```python
from build123d import *

# Parameters (mm, degrees)
F0_W = 2.2650395424
F0_H = 3.0083153293


with BuildPart() as f1:
    # F0 (on Front) → F1 (revolve)
    with BuildSketch(Plane.XZ):
        Polygon((-45.5736112406, 22.732421128), (-30.0700433831, 13.9608631497), (-22.3959553987, 18.4812154621), (-14.7995633587, 31.907699076), (-14.8772593031, 40.8138303776), (-30.3808271606, 40.8138303776), (-30.3808271606, 49.5853883559), (-45.7290031294, 40.5446837311), (-45.6866675821, 35.6918442891), (-41.150290519, 35.6918442891), (-41.150290519, 27.58526057), (-45.615946788, 27.58526057), align=None)
        Polygon((-50.1523238511, 27.58526057), (-45.615946788, 27.58526057), (-45.6866675821, 35.6918442891), (-50.1523238511, 35.6918442891), (-50.1523238511, 33.1427100942), (-47.8872843087, 33.1427100942), (-47.8872843087, 30.1343947649), (-50.1523238511, 30.1343947649), align=None)
        Polygon((-45.6866675821, 35.6918442891), (-45.615946788, 27.58526057), (-41.150290519, 27.58526057), (-41.150290519, 35.6918442891), align=None)
        with Locations((-51.2848436223, 31.6385524296)):
            Rectangle(F0_W, F0_H)
        with Locations((-49.0198040799, 31.6385524296)):
            Rectangle(F0_W, F0_H)
    revolve(axis=Axis((0.4552025348, 0, 0), (1, 0, 0)))


solid = f1.part
```
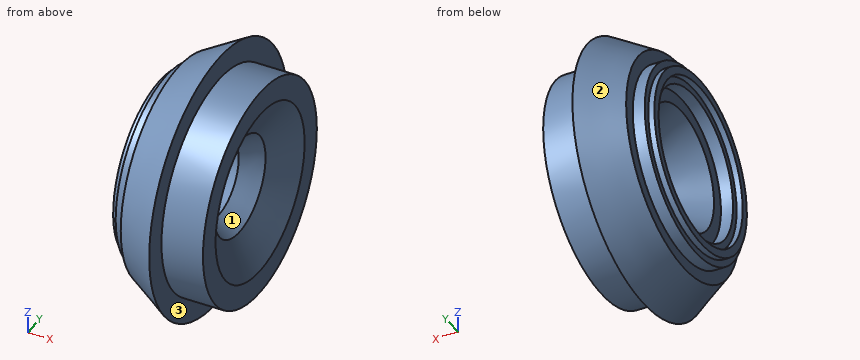
Read the model definition and answer for the solid it produces. Units are mm, in the model's axes. Face numbers are marked on the shaded views. Round coordinates to 2 decimals unless told otherwise and drop trailing zeros. Write each loop counter-clockwise with the first axis right and the second up, starting at its lowest first coordinate (ties: lowest second). Pieces come first, ordered by that corner, then holes. Notation, with made-up numbers: (-13, 16) -> (6, 16) arc R32 ccw to (6, 52) -> close; hole circle Ø10 at (-28.5, 12). An arc over 180 degrees is marked (long way). Answer in a Markdown table with one row per item. Add a question column.
1) Consider line 1 (Y direction, x = -51, z = 0); line 2 (Y direction, x = -46.85, z = 0). Determine where each line is inside the solid, lowest interval first.
2) Given P1, Ø2, axis at y = -12.5, z = -33, coming from the +X side; P2, Ø2, axis at x = -41, z = -28.5, coming from the -Y side; P3, Ø1, axis at y = 21, z = 23, coming from the +X side; P4, Ø10, axis at y = 1, z = 6.5, coming from the -X side, each flat-ended and moving along its own axis, determine where each tip first touches the part or whether it passes through.
3) Find section B-B, the plane x = -47. Determine the outline of the cut face in (y, z).
4) Find section D-D, the plane x = -34. Determine the outline of the cut face in (y, z).
5) Determine the mould class of the marked faces 1, 2 and 3 for opening direction Y: pulls with the +Y half, pulls with the -Y half, needs draft (parallel to the pull), parting line crosses it, or undercut.
Findings below:
| question | item | result |
|---|---|---|
| 1 | line 1 | -33.14 to -30.13, 30.13 to 33.14 |
| 1 | line 2 | -35.69 to -27.59, 27.59 to 35.69 |
| 2 | P1 | x = -14.82 |
| 2 | P2 | y = -33.78 |
| 2 | P3 | x = -14.95 |
| 2 | P4 | through |
| 3 | outline | circle Ø71.38 at (0, 0); hole circle Ø55.17 at (0, 0) |
| 4 | outline | circle Ø94.91 at (0, 0); hole circle Ø32.37 at (0, 0) |
| 5 | face 1 | undercut |
| 5 | face 2 | parting line crosses it |
| 5 | face 3 | needs draft |
